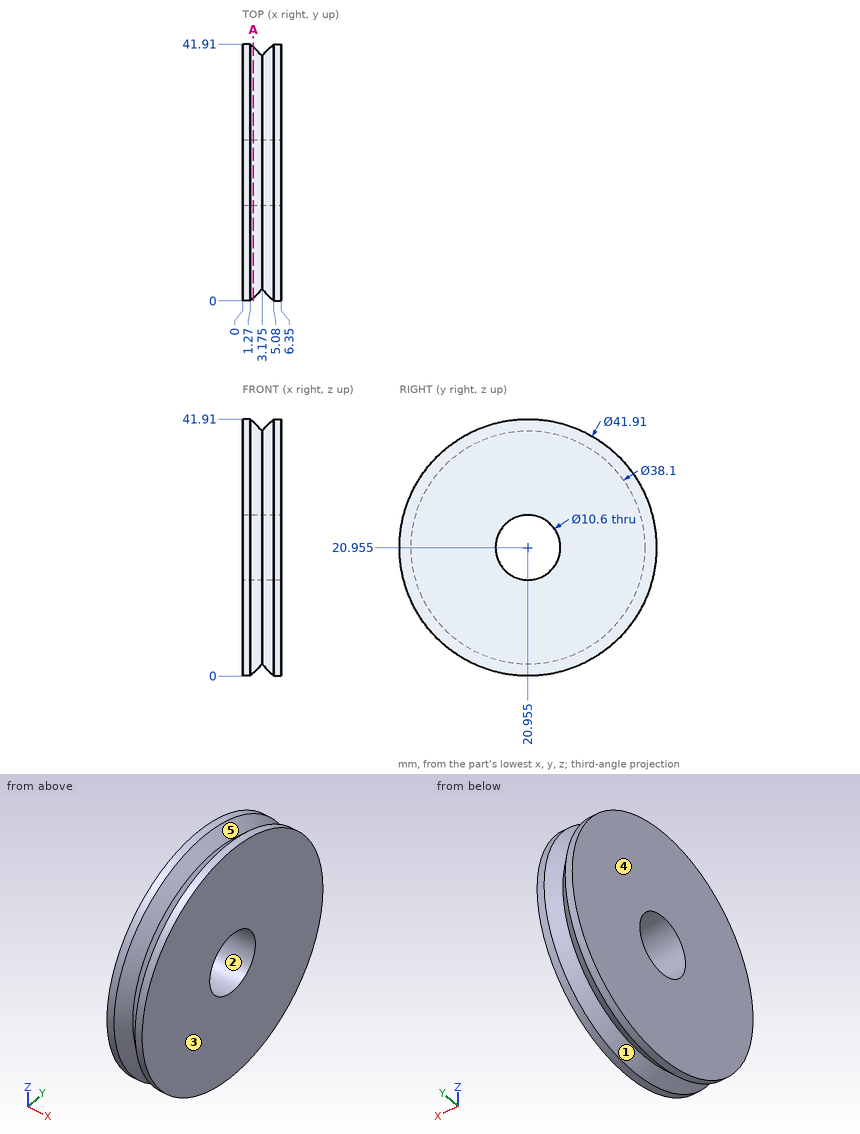
For this review, use the dimensioned drawing (mm, ordinates from the lowest corner) and the shaded views. A direction names the side the tool comes from. Coordinates: 2 decimals unless noted, no trailing zeros. Order: outer loops, then holes, each group sorted by start corner. A loop starts at its lowest first (then second) coordinate and runs counter-clockwise, first axis right, second up. Notation, with made-up numbers: (81.25, 42.5) -> (103.25, 42.5) arc R21 cw to (103.25, 59.5) -> close; hole circle Ø1 at (59.5, 13.25). An arc over 180 degrees is marked (long way). One line per item, written item: value. Start each with the question number.
Q1. For probe 1 along Z at (x, y) = (5.25, 22.5); probe 2 along Z at (x, y) = (4.25, 19.5); probe 3 along X at (y, z) = (31, 4), list the stretches that pass through material, from the lowest coordinate up.
Q2. Insertion check: pin 1 Ø1 at (x, y) = (1.5, 19.5) entering from -Z; pin 2 Ø3 at (x, z) = (3, 33) entering from -Y; pin 3 Ø1.5 at (x, z) = (1, 24.5) entering from +Y; pin 4 Ø8.5 at (y, z) = (20.955, 20.955) entering from -X. Each pin has a flat end and moves straight along its axis. Give the tip position at first contact, or say it passes through.
Q3. Tool access review of the marked faces 4 and 5: name each direction out of +Z, -Z, +X, -X, +Y, -Y from which nothing blocks a thin tool from reaching the whole face with its end or side.
Q4. Take a section at A-A, the plane x = 1.75. State the section outline as (y, z) points (3 decimals).
Q5. Mouldability with a two-part tool opening along X and no side actions: class the marked faces 1, 2 and 3 as pulls with the +X half, pulls with the -X half, needs draft (parallel to the pull), parting line crosses it, or undercut.
Values follow:
1. probe 1: z = 0.06 to 15.89, 26.02 to 41.85
1. probe 2: z = 0.88 to 15.86, 26.05 to 41.03
1. probe 3: x = 0 to 2.52, 3.83 to 6.35
2. pin 1: stops at z = 0.02
2. pin 2: stops at y = 3.82
2. pin 3: stops at y = 41.72
2. pin 4: passes through
3. face 4: +Z, -Z, -X, +Y, -Y
3. face 5: none
4. outline: circle Ø40.95 at (20.955, 20.955); hole circle Ø10.6 at (20.955, 20.955)
5. face 1: undercut
5. face 2: needs draft
5. face 3: pulls with the +X half
